```python
from build123d import *

# Parameters (mm, degrees)
F1_DEPTH = 3.2258
F2_W     = 25.4
F2_H     = 10.16
F3_DEPTH = 3.3782
F5_DEPTH = 2.54
F7_DEPTH = 3.2268


with BuildPart() as f1:
    # F0 (on Top) → F1 (new body)
    with BuildSketch(Plane.XY):
        with BuildLine():
            Line((46.99, 18.161), (-46.99, 18.161))
            Line((-46.99, 18.161), (-46.99, 4.441107))
            ThreePointArc((-46.99, 4.441107), (-40.364333, -6.077512), (-49.784, -14.189891))
            Line((-49.784, -14.189891), (-49.784, -16.475891))
            ThreePointArc((-49.784, -16.475891), (-39.920006, -11.161147), (-38.933262, 0))
            Line((-38.933262, 0), (-10.16, 0))
            Line((-10.16, 0), (-10.16, 3.937))
            Line((-10.16, 3.937), (10.16, 3.937))
            Line((10.16, 3.937), (10.16, 0))
            Line((10.16, 0), (38.933262, 0))
            ThreePointArc((38.933262, 0), (39.920006, -11.161147), (49.784, -16.475891))
            Line((49.784, -16.475891), (49.784, -14.189891))
            ThreePointArc((49.784, -14.189891), (40.364333, -6.077512), (46.99, 4.441107))
            Line((46.99, 4.441107), (46.99, 18.161))
        make_face()
    extrude(amount=F1_DEPTH)

    # F2 (on face) → F3 (join)
    with BuildSketch(Plane.XY.offset(3.2258)):
        with Locations((-34.29, 13.081)):
            Rectangle(F2_W, F2_H)
    extrude(amount=F3_DEPTH)

    # F4 (on face) → F5 (cut)
    with BuildSketch(Plane(origin=(0, 0, 0), x_dir=(1, 0, 0), z_dir=(0, 0, -1))):
        with BuildLine():
            Line((-46.99, -6.820624), (-46.99, -16.077196))
            ThreePointArc((-46.99, -16.077196), (-42.60338, -11.44891), (-46.99, -6.820624))
        make_face()
        with BuildLine():
            ThreePointArc((46.99, -6.820624), (42.60338, -11.44891), (46.99, -16.077196))
            Line((46.99, -16.077196), (46.99, -6.820624))
        make_face()
    extrude(amount=-F5_DEPTH, mode=Mode.SUBTRACT)

    # F6 (on face) → F7 (cut, through all)
    with BuildSketch(Plane.XY.offset(3.2258)):
        with BuildLine():
            Line((-48.518732, -16.407924), (-48.518732, -14.10548))
            ThreePointArc((-48.518732, -14.10548), (-49.149959, -14.168765), (-49.784, -14.189891))
            Line((-49.784, -14.189891), (-49.784, -16.475891))
            ThreePointArc((-49.784, -16.475891), (-49.150454, -16.458887), (-48.518732, -16.407924))
        make_face()
        with BuildLine():
            ThreePointArc((48.518732, -16.407924), (49.150454, -16.458887), (49.784, -16.475891))
            Line((49.784, -16.475891), (49.784, -14.189891))
            ThreePointArc((49.784, -14.189891), (49.149959, -14.168765), (48.518732, -14.10548))
            Line((48.518732, -14.10548), (48.518732, -16.407924))
        make_face()
    extrude(amount=-F7_DEPTH, mode=Mode.SUBTRACT)


solid = f1.part
```
Work out the finished part from the listing and answer in its coordinate system (mm). A direction names the side the tool comes from. Round coordinates to 2 decimals unless told otherwise and drop trailing zeros. Write each loop counter-clockwise with the first axis right and the second up, starting at its lowest first coordinate (ties: lowest second). Pieces come first, ordered by that corner, then holes.
1) A cutting plane is placed at B-B on x = -27. Determine the outline of the cut face in (y, z), and give its area (3 significant figures).
2) Determine the mould class of faces 1 (the face through (0, 3.937, 2)), 2 (the face through (45, 11, 2.54)), 3 (the face through (46.99, 10, 3)) for opening direction Y: pulls with the +Y half, pulls with the -Y half, needs draft (parallel to the pull), parting line crosses it, or undercut.
3) Which of the six approach directions +Z, -Z, +X, -X, +Y, -Y give full straight-line access (tool end or side, diameter ignored) to faces 4 (the face through (-48.519, -15, 2)), 5 (the face through (-34, 8.001, 5)), 6 (the face through (-45, 11, 2.54)), 7 (the face through (-46.99, 11, 4)), 8 (the face through (-21.59, 13, 5))?
4) A cutting plane is placed at A-A on z = 1.25. Determine the outline of the cut face in (x, y) (3 decimals), and give its area (3 significant figures).
5) Consider probe 1 along Z at (x, y) = (-40, 7); probe 2 along Y at (x, z) = (15.5, 1.25); probe 3 along X at (y, z) = (-10, 2.25). Determine where each line is inside the solid, lowest interval first.
6) Flat-ended cylindrical pins translate along their axes: P1, Ø1, axis at x = -31, z = 1, coming from the -Y side; P2, Ø3.5, axis at y = 10.5, z = 3, coming from the -X side; P3, Ø2.5, axis at y = 13, z = 5, coming from the +X side; P4, Ø8, axis at x = -23, y = -6.5, coming from the +Z side. Find the tip coordinate at first contact, or state that the pin passes through.
7) A cutting plane is placed at C-C on y = -7.5. Determine the outline of the cut face in (x, z), and give its area (3 significant figures).
8) A cutting plane is placed at D-D on y = 14.5. Determine the outline of the cut face in (x, z).
Entries:
1. outline: (0, 0) - (18.16, 0) - (18.16, 6.6) - (8, 6.6) - (8, 3.23) - (0, 3.23) - close
1. area: 92.9 mm2
2. face 1: pulls with the -Y half
2. face 2: undercut
2. face 3: needs draft
3. face 4: +Z, -Z, -X, +Y, -Y
3. face 5: +Z, +X, -X, -Y
3. face 6: -Z, -X
3. face 7: +Z, -Z, -X, +Y
3. face 8: +Z, +X, +Y, -Y
4. outline: (-48.519, -16.408) arc R11.811 ccw to (-38.933, 0) - (-10.16, 0) - (-10.16, 3.937) - (10.16, 3.937) - (10.16, 0) - (38.933, 0) arc R11.811 ccw to (48.519, -16.408) - (48.519, -14.105) arc R9.525 cw to (46.99, 4.441) - (46.99, 6.821) arc R4.635 cw to (46.99, 16.077) - (46.99, 18.161) - (-46.99, 18.161) - (-46.99, 16.077) arc R4.635 cw to (-46.99, 6.821) - (-46.99, 4.441) arc R9.525 cw to (-48.519, -14.105) - close
4. area: 1,630 mm2
5. probe 1: z = 0 to 3.23
5. probe 2: y = 0 to 18.16
5. probe 3: x = -41.89 to -39.25, 39.25 to 41.89
6. P1: stops at y = 0
6. P2: stops at x = -46.99
6. P3: stops at x = -21.59
6. P4: passes through
7. outline: (-40.69, 0) - (-38.32, 0) - (-38.32, 3.23) - (-40.69, 3.23) - close; (38.32, 0) - (40.69, 0) - (40.69, 3.23) - (38.32, 3.23) - close
7. area: 15.3 mm2
8. outline: (-46.99, 2.54) - (-43.75, 2.54) - (-43.75, 0) - (43.75, 0) - (43.75, 2.54) - (46.99, 2.54) - (46.99, 3.23) - (-21.59, 3.23) - (-21.59, 6.6) - (-46.99, 6.6) - close
